For this review, take the finished solid that the model builds, in its own axes (mm). Face numbers are marked on the shaded views. A direction names the side the tool comes from. Round coordinates to 2 decimals unless told otherwise and drop trailing zeros. Loops run counter-clockwise (first coordinate to the right, second up) from the corner with the lowest first, then second, coordinate; pieces in that order, holes last.
1. Clearance check with flat-ended pins moving along their axes: pin 1 Ø5 at (x, z) = (-1.5, -2) entering from -Y; pin 2 Ø0.9 at (x, y) = (0, 2.5) entering from +Z. State where each tip first meets the part, or that it passes through.
2. Tool access review of the marked faces 5, 6 and 7: name each direction out of +Z, -Z, +X, -X, +Y, -Y from which nothing blocks a thin tool from reaching the whole face with its end or side.
3. Consider section B-B on x = -5. State the section outline as (y, z) points, then the cut area to 3 significant figures.
4. To check wall thickness, follow line 1 along Y through (x, z) = (3, -4.5); line 2 along Z through (x, y) = (-4.75, -2.75); line 3 along X through (y, z) = (-2.5, 1). State the ranges of each line that lie inside material, in increasing order.
5. Draft analysis for pull direction X (two halves, no side actions). For the marked faces 1, 2, 3 and 4, state which applies: released by +X, released by -X, zero draft, split by the parting line, or undercut.
6. Consider section A-A on x = 7.25. State the section outline as (y, z) points.
from build123d import *

# Parameters (mm, degrees)
F0_W      = 24.1
F0_H      = 10.1
F1_DEPTH  = 3.1
F2_W      = 1.1417344213
F2_H      = 2.2121103248
F2_W_2    = 1.0703755543
F2_H_2    = 2.1407519816
F2_W_3    = 1.0703760199
F2_R      = 0.9384971682
F3_DEPTH  = 0.2
F4_R      = 1
F5_R      = 1
F6_R      = 1
F7_R      = 1
F8_W      = 10.8690736815
F8_H      = 10.1
F9_DEPTH  = 0.1
F10_W     = 6.1270436272
F10_H     = 1.7071549356
F11_DEPTH = 0.1


with BuildPart() as f1:
    # F0 (on Front) → F1 (new body, symmetric)
    with BuildSketch(Plane.XZ):
        Rectangle(F0_W, F0_H)
    extrude(amount=F1_DEPTH, both=True)

    # F2 (on face) → F3 (join)
    with BuildSketch(Plane.XY.offset(5.05)):
        with Locations((-10.5197010562, 0.0642262748)):
            Rectangle(F2_W, F2_H)
        with Locations((-8.4859863855, 0.0999054464)):
            Rectangle(F2_W_2, F2_H_2)
        with Locations((-6.4165925141, 0.0642262748)):
            Rectangle(F2_W_3, F2_H)
        with Locations((6.4165925141, 0.0642262748)):
            Rectangle(F2_W_3, F2_H)
        with Locations((8.4859863855, 0.0999054464)):
            Rectangle(F2_W_2, F2_H_2)
        with Locations((10.5197010562, 0.0642262748)):
            Rectangle(F2_W, F2_H)
        Circle(F2_R)
    extrude(amount=F3_DEPTH)

    # F4
    f4_edges = [f1.edges().sort_by_distance(p)[0] for p in [
        (-12.05, 3.1, 0),
    ]]
    fillet(f4_edges, radius=F4_R)

    # F5
    f5_edges = [f1.edges().sort_by_distance(p)[0] for p in [
        (-12.05, -3.1, 0),
    ]]
    fillet(f5_edges, radius=F5_R)

    # F6
    f6_edges = [f1.edges().sort_by_distance(p)[0] for p in [
        (12.05, 3.1, 0),
    ]]
    fillet(f6_edges, radius=F6_R)

    # F7
    f7_edges = [f1.edges().sort_by_distance(p)[0] for p in [
        (12.05, -3.1, 0),
    ]]
    fillet(f7_edges, radius=F7_R)

    # F8 (on face) → F9 (cut)
    with BuildSketch(Plane.XZ.offset(3.1)):
        with Locations((-0.0399495475, 0)):
            Rectangle(F8_W, F8_H)
    extrude(amount=-F9_DEPTH, mode=Mode.SUBTRACT)

    # F10 (on face) → F11 (join)
    with BuildSketch(Plane.XY.offset(5.05)):
        with Locations((-0.3709765151, 2.2464225322)):
            Rectangle(F10_W, F10_H)
        with BuildLine():
            add(Edge.make_bspline(
                [(-1.9910920446, 2.7120085217), (-1.9402540003, 2.5879636937), (-1.9402540003, 2.4193169547)],
                knots=[0, 0, 0, 1, 1, 1], degree=2))
            add(Edge.make_bspline(
                [(-1.9402540003, 2.4193169547), (-1.9402540003, 1.6921295692), (-2.5028616905, 1.6921295692)],
                knots=[0, 0, 0, 1, 1, 1], degree=2))
            add(Edge.make_bspline(
                [(-2.5028616905, 1.6921295692), (-2.6012841443, 1.6921295692), (-2.6587650264, 1.709211152)],
                knots=[0, 0, 0, 1, 1, 1], degree=2))
            Line((-2.6587650264, 1.709211152), (-2.6587650264, 1.8304090496))
            add(Edge.make_bspline(
                [(-2.6587650264, 1.8304090496), (-2.5909809673, 1.8084470145), (-2.5047596442, 1.8084470145)],
                knots=[0, 0, 0, 1, 1, 1], degree=2))
            add(Edge.make_bspline(
                [(-2.5047596442, 1.8084470145), (-2.301407467, 1.8084470145), (-2.1975622885, 1.9342542281)],
                knots=[0, 0, 0, 1, 1, 1], degree=2))
            add(Edge.make_bspline(
                [(-2.1975622885, 1.9342542281), (-2.0937171101, 2.0600614417), (-2.084498478, 2.3200810923)],
                knots=[0, 0, 0, 1, 1, 1], degree=2))
            Line((-2.084498478, 2.3200810923), (-2.0945305188, 2.3200810923))
            add(Edge.make_bspline(
                [(-2.0945305188, 2.3200810923), (-2.1411659514, 2.2498568071), (-2.2183042106, 2.212982279)],
                knots=[0, 0, 0, 1, 1, 1], degree=2))
            add(Edge.make_bspline(
                [(-2.2183042106, 2.212982279), (-2.2954424698, 2.1761077508), (-2.3919669699, 2.1761077508)],
                knots=[0, 0, 0, 1, 1, 1], degree=2))
            add(Edge.make_bspline(
                [(-2.3919669699, 2.1761077508), (-2.5562755291, 2.1761077508), (-2.6529355973, 2.2743946365)],
                knots=[0, 0, 0, 1, 1, 1], degree=2))
            add(Edge.make_bspline(
                [(-2.6529355973, 2.2743946365), (-2.7495956655, 2.3726815221), (-2.7495956655, 2.5489200756)],
                knots=[0, 0, 0, 1, 1, 1], degree=2))
            add(Edge.make_bspline(
                [(-2.7495956655, 2.5489200756), (-2.7495956655, 2.7419690758), (-2.6415478754, 2.8538127733)],
                knots=[0, 0, 0, 1, 1, 1], degree=2))
            add(Edge.make_bspline(
                [(-2.6415478754, 2.8538127733), (-2.5335000852, 2.9656564707), (-2.3572615317, 2.9656564707)],
                knots=[0, 0, 0, 1, 1, 1], degree=2))
            add(Edge.make_bspline(
                [(-2.3572615317, 2.9656564707), (-2.2309120456, 2.9656564707), (-2.1364210673, 2.9008549103)],
                knots=[0, 0, 0, 1, 1, 1], degree=2))
            add(Edge.make_bspline(
                [(-2.1364210673, 2.9008549103), (-2.0419300889, 2.8360533498), (-1.9910920446, 2.7120085217)],
                knots=[0, 0, 0, 1, 1, 1], degree=2))
        make_face(mode=Mode.SUBTRACT)
        Polygon((-1.2990168017, 2.4098271865), (-0.7822311354, 1.709211152), (-0.9516912831, 1.709211152), (-1.4031331164, 2.3100490515), (-1.5330073735, 2.1948161511), (-1.5330073735, 1.709211152), (-1.676980715, 1.709211152), (-1.676980715, 2.9480326154), (-1.5330073735, 2.9480326154), (-1.5330073735, 2.3336379041), (-0.9712130921, 2.9480326154), (-0.8009395357, 2.9480326154), align=None, mode=Mode.SUBTRACT)
        with BuildLine():
            Line((0.1168566239, 1.8396276817), (0.1168566239, 1.709211152))
            Line((0.1168566239, 1.709211152), (-0.6973654935, 1.709211152))
            Line((-0.6973654935, 1.709211152), (-0.6973654935, 1.8304090496))
            Line((-0.6973654935, 1.8304090496), (-0.3711886013, 2.1582127592))
            add(Edge.make_bspline(
                [(-0.3711886013, 2.1582127592), (-0.2220636714, 2.3092356428), (-0.17461483, 2.3736304989)],
                knots=[0, 0, 0, 1, 1, 1], degree=2))
            add(Edge.make_bspline(
                [(-0.17461483, 2.3736304989), (-0.1271659887, 2.438025355), (-0.103441568, 2.4990310082)],
                knots=[0, 0, 0, 1, 1, 1], degree=2))
            add(Edge.make_bspline(
                [(-0.103441568, 2.4990310082), (-0.0797171473, 2.5600366613), (-0.0797171473, 2.6302609465)],
                knots=[0, 0, 0, 1, 1, 1], degree=2))
            add(Edge.make_bspline(
                [(-0.0797171473, 2.6302609465), (-0.0797171473, 2.729496809), (-0.1399093918, 2.7875199635)],
                knots=[0, 0, 0, 1, 1, 1], degree=2))
            add(Edge.make_bspline(
                [(-0.1399093918, 2.7875199635), (-0.2001016362, 2.8455431181), (-0.3069293133, 2.8455431181)],
                knots=[0, 0, 0, 1, 1, 1], degree=2))
            add(Edge.make_bspline(
                [(-0.3069293133, 2.8455431181), (-0.3839320044, 2.8455431181), (-0.4530717446, 2.8200563119)],
                knots=[0, 0, 0, 1, 1, 1], degree=2))
            add(Edge.make_bspline(
                [(-0.4530717446, 2.8200563119), (-0.5222114849, 2.7945695057), (-0.6068059906, 2.7275988553)],
                knots=[0, 0, 0, 1, 1, 1], degree=2))
            Line((-0.6068059906, 2.7275988553), (-0.6813684555, 2.8233099467))
            add(Edge.make_bspline(
                [(-0.6813684555, 2.8233099467), (-0.5102814905, 2.9656564707), (-0.3085561307, 2.9656564707)],
                knots=[0, 0, 0, 1, 1, 1], degree=2))
            add(Edge.make_bspline(
                [(-0.3085561307, 2.9656564707), (-0.1339443946, 2.9656564707), (-0.0348441003, 2.8763170809)],
                knots=[0, 0, 0, 1, 1, 1], degree=2))
            add(Edge.make_bspline(
                [(-0.0348441003, 2.8763170809), (0.0642561941, 2.7869776911), (0.0642561941, 2.6362259437)],
                knots=[0, 0, 0, 1, 1, 1], degree=2))
            add(Edge.make_bspline(
                [(0.0642561941, 2.6362259437), (0.0642561941, 2.518281681), (-0.0019010476, 2.4030487806)],
                knots=[0, 0, 0, 1, 1, 1], degree=2))
            add(Edge.make_bspline(
                [(-0.0019010476, 2.4030487806), (-0.0680582892, 2.2878158802), (-0.249177295, 2.1115773266)],
                knots=[0, 0, 0, 1, 1, 1], degree=2))
            Line((-0.249177295, 2.1115773266), (-0.5203135312, 1.8464060876))
            Line((-0.5203135312, 1.8464060876), (-0.5203135312, 1.8396276817))
            Line((-0.5203135312, 1.8396276817), (0.1168566239, 1.8396276817))
        make_face(mode=Mode.SUBTRACT)
    extrude(amount=F11_DEPTH)


solid = f1.part
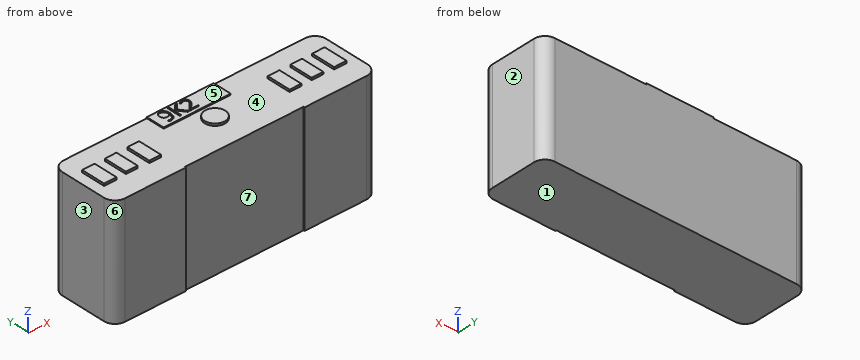
Resolved:
1. pin 1: stops at y = -3
1. pin 2: stops at z = 5.15
2. face 5: +Z, +X, -X, +Y
2. face 6: +Z, -Z, -X, -Y
2. face 7: +Z, -Z, -Y
3. outline: (-3, -5.05) - (3.1, -5.05) - (3.1, 5.05) - (-3, 5.05) - close
3. area: 61.6 mm2
4. line 1: y = -3 to 3.1
4. line 2: z = -5.05 to 5.05
4. line 3: x = -11.97 to 11.97
5. face 1: zero draft
5. face 2: released by +X
5. face 3: released by -X
5. face 4: undercut
6. outline: (-3.1, -5.05) - (3.1, -5.05) - (3.1, 5.05) - (-3.1, 5.05) - close
